The model under review builds one solid part; all positions refer to its coordinate system, in mm. Round coordinates to 2 decimals unless told otherwise and drop trailing zeros. Write each loop counter-clockwise with the first axis right and the second up, starting at its lowest first coordinate (ties: lowest second). Pieces come first, ordered by that corner, then holes. Notation, with made-up numbers: (63.25, 76.5) -> (122.25, 76.5) arc R19 ccw to (122.25, 100.5) -> close; hole circle Ø11 at (76.25, 86.25). An arc over 180 degrees is marked (long way). Use CSV: the item, a comma, the result in double quotes. Start each with the question number.
1) For pin 1 Ø1.9 at (x, z) = (-50, -92.76) entering from +Y, flat-tipped, find the tip position at first contact; note if it passes through.
2) Take a section at C-C, the plane z = -55. Give the boundary of the cut face in (x, y), then the cut area to 3 significant figures.
3) Take a section at B-B, the plane x = -13. Give the boundary of the cut face in (y, z), then the cut area to 3 significant figures.
4) Wall thickness on probe 1 along Z at (x, y) = (22.5, -1.15); probe 2 along X at (y, z) = (-0.75, -133.76); probe 3 along Z at (x, y) = (-3, -2.4): over which ranges is each line inside the solid? List them lowest first. Write a range as [from, to].
5) Take a section at A-A, the plane x = 22.5. Give the boundary of the cut face in (y, z), then the cut area to 3 significant figures.
6) Take a section at D-D, the plane y = -0.95. State how many separate pieces and enclosed holes the cut face has, then the cut area to 3 significant figures.
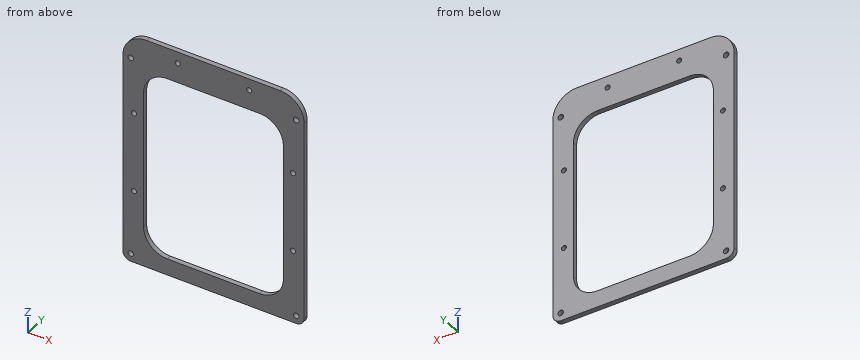
Solid Edge part; units mm, degrees
sketch "Sketch1" plane through (0, 0, 0) normal (0, -1, 0) x (1, 0, 0)
  line L0 (-57, -7.76) -> (-57, -133.76)
  arc A0 (-52, -138.76) -> (-57, -133.76) centre (-52, -133.76) cw
  line L1 (-52, -138.76) -> (52, -138.76)
  arc A1 (57, -133.76) -> (52, -138.76) centre (52, -133.76) cw
  line L2 (57, -133.76) -> (57, -7.76)
  arc A2 (42, 7.24) -> (57, -7.76) centre (42, -7.76) cw
  line L3 (42, 7.24) -> (-42, 7.24)
  arc A3 (-42, 7.24) -> (-57, -7.76) centre (-42, -7.76) ccw
  circle A4 centre (-52, -7.76) radius 1.75
  circle A5 centre (-22.5, 0) radius 1.6
  circle A6 centre (22.5, 0) radius 1.6
  circle A7 centre (52, -7.76) radius 1.75
  circle A8 centre (-52, -133.76) radius 1.75
  circle A9 centre (52, -133.76) radius 1.75
  line L4 (-29, -12.4008) -> (29, -12.4008)
  arc A10 (29, -12.4008) -> (44, -27.4008) centre (29, -27.4008) cw
  line L5 (44, -27.4008) -> (44, -113.4008)
  arc A11 (44, -113.4008) -> (29, -128.4008) centre (29, -113.4008) cw
  line L6 (29, -128.4008) -> (-29, -128.4008)
  arc A12 (-29, -128.4008) -> (-44, -113.4008) centre (-29, -113.4008) cw
  line L7 (-44, -113.4008) -> (-44, -27.4008)
  arc A13 (-29, -12.4008) -> (-44, -27.4008) centre (-29, -27.4008) ccw
  circle A14 centre (-50, -42.76) radius 1.6
  circle A15 centre (-50, -92.76) radius 1.6
  circle A16 centre (50, -42.76) radius 1.6
  circle A17 centre (50, -92.76) radius 1.6
extrude "Protrusion1" add sketch "Sketch1" along normal blind 3
properties material "ABS Plastic, medium impact"
Values found:
1,pin 1,"through"
2,outline,"(-57, -3) -> (-44, -3) -> (-44, 0) -> (-57, 0) -> close; (44, -3) -> (57, -3) -> (57, 0) -> (44, 0) -> close"
2,area,"78.0 mm²"
3,outline,"(-3, -138.76) -> (0, -138.76) -> (0, -128.4) -> (-3, -128.4) -> close; (-3, -12.4) -> (0, -12.4) -> (0, 7.24) -> (-3, 7.24) -> close"
3,area,"90.0 mm²"
4,probe 1,"[-138.76, -128.4], [-12.4, -1.6], [1.6, 7.24]"
4,probe 2,"[-57, -53.75], [-50.25, 50.25], [53.75, 57]"
4,probe 3,"[-138.76, -128.4], [-12.4, 7.24]"
5,outline,"(-3, -138.76) -> (0, -138.76) -> (0, -128.4) -> (-3, -128.4) -> close; (-3, -12.4) -> (0, -12.4) -> (0, -1.6) -> (-3, -1.6) -> close; (-3, 1.6) -> (0, 1.6) -> (0, 7.24) -> (-3, 7.24) -> close"
5,area,"80.4 mm²"
6,separate pieces,"1"
6,enclosed holes,"11"
6,area,"6,440 mm²"
